Here's how the part is built. I have some questions about the finished solid (model axes, mm). A direction names the side the tool comes from. Give positions to 0.01 mm unless a question says otherwise; leave off trailing zeros. Loops run counter-clockwise (first coordinate to the right, second up) from the corner with the lowest first, then second, coordinate; pieces in that order, holes last. Notation, with made-up numbers: (-32.75, 37) - (-23.75, 37) arc R22 ccw to (-23.75, 49) - close; hole circle Ø3 at (9.25, 76.5). An arc over 180 degrees is marked (long way). Return JSON: item names as keys, results as strings. Group by question number.
(1) If we section it at B-B (y = 72): Please give me the cut outline in (x, z), then the cut area to 3 significant figures.
(2) If we section it at D-D (z = 0.8): State how many separate pieces and enclosed holes the cut face has, then the cut area to 3 significant figures.
(3) On a 3-axis mill with a long thin cutter (end or side, diameter ignored), from which of +Z, -Z, +X, -X, +Y, -Y can I reach the whole of each face in a straight line? I mean faces 4 (the flat face through (1, 0, 1)), 5 (the cylindrical face through (-46.1, 84.5, 1.5)). Say none if no direction works.
(4) If we section it at A-A (x = 25): Please give me the cut outline in (y, z), then the cut area to 3 significant figures.
(5) If we mould it in two halves opening along X, with no side actions, what happens to faces 1 (the cylindrical face through (45.9, 29.5, 1.5)), 2 (the flat face through (-56, 71, 1)), 3 (the flat face through (1, 145, 1))? For each: released by +X, released by -X, zero draft, split by the parting line, or undercut.
(6) For P1, Ø2.5, axis at x = -25, y = 45, coming from the -Z side, with a flat end and sliding along its axis, tell me the tip position at first contact or that it passes through.
(7) If we section it at C-C (x = -46): Please give me the cut outline in (y, z).
(8) I need wall thicknesses on probe 1 along Y at (x, z) = (-25, 0.95); probe 2 along X at (y, z) = (49.5, 1.1); probe 3 along X at (y, z) = (69, 1.4). Which ranges of each line are inside material? Lowest first, please. Write a range as [from, to].
```python
from build123d import *

# Parameters (mm, degrees)
F0_W     = 56
F0_H     = 145
F1_DEPTH = 3
F3_D     = 3
F8_DEPTH = 25
F11_D    = 3
F13_D    = 3


with BuildPart() as f1:
    # F0 (on Top) → F1 (new body)
    with BuildSketch(Plane.XY):
        with Locations((28, 72.5)):
            Rectangle(F0_W, F0_H)
    extrude(amount=F1_DEPTH)

    # F3 (through all)
    with Locations(Plane.XY.offset(3)):
        with Locations((25, 69), (25, 45)):
            Hole(F3_D / 2)

    # F7 (on face) → F8 (cut)
    with BuildSketch(Plane.XY.offset(3)):
        with BuildLine():
            ThreePointArc((48.5, 82), (46, 84.5), (43.5, 82))
            Line((43.5, 82), (43.5, 32))
            ThreePointArc((43.5, 32), (46, 29.5), (48.5, 32))
            Line((48.5, 32), (48.5, 82))
        make_face()
    extrude(amount=-F8_DEPTH, mode=Mode.SUBTRACT)

    # F11 (through all)
    with Locations(Plane.XY.offset(3)):
        with Locations((12, 133)):
            Hole(F11_D / 2)

    # F13 (through all)
    with Locations(Plane.XY.offset(3)):
        with Locations((30, 22.5)):
            Hole(F13_D / 2)

    # F14: F1 across plane


with BuildPart() as f1_1:
    add(f1.part)
    add(f1.part.mirror(Plane.YZ))


solid = f1_1.part
```
Values:
{
 "1": {"outline": "(-56, 0) - (-48.5, 0) - (-48.5, 3) - (-56, 3) - close; (-43.5, 0) - (43.5, 0) - (43.5, 3) - (-43.5, 3) - close; (48.5, 0) - (56, 0) - (56, 3) - (48.5, 3) - close", "area": "306 mm2"},
 "2": {"separate pieces": "1", "enclosed holes": "10", "area": "15,600 mm2"},
 "3": {"face 4": "+Z, -Z, +X, -X, -Y", "face 5": "+Z, -Z"},
 "4": {"outline": "(0, 0) - (43.5, 0) - (43.5, 3) - (0, 3) - close; (46.5, 0) - (67.5, 0) - (67.5, 3) - (46.5, 3) - close; (70.5, 0) - (145, 0) - (145, 3) - (70.5, 3) - close", "area": "417 mm2"},
 "5": {"face 1": "undercut", "face 2": "released by -X", "face 3": "zero draft"},
 "6": {"P1": "through"},
 "7": {"outline": "(0, 0) - (29.5, 0) - (29.5, 3) - (0, 3) - close; (84.5, 0) - (145, 0) - (145, 3) - (84.5, 3) - close"},
 "8": {"probe 1": "[0, 43.5], [46.5, 67.5], [70.5, 145]", "probe 2": "[-56, -48.5], [-43.5, 43.5], [48.5, 56]", "probe 3": "[-56, -48.5], [-43.5, -26.5], [-23.5, 23.5], [26.5, 43.5], [48.5, 56]"}
}
